```python
from build123d import *

# Parameters (mm, degrees)
F1_DEPTH = 20
F3_D     = 6
F4_SIZE  = 2
F5_R     = 2
F7_D     = 12
F7_DEPTH = 12
F7_TIP   = 3.6051637142
F9_D     = 12
F9_DEPTH = 12
F9_TIP   = 3.6051637142


# Not quite as in the source:
# - a feature names something its author has since deleted; it is built from what else it names


with BuildPart() as f1:
    # F0 (on Top) → F1 (new body)
    with BuildSketch(Plane.XY):
        with BuildLine():
            Line((0, 18), (0, 22.5))
            Line((0, 22.5), (0, 37.4649850279))
            Line((0, 37.4649850279), (-7, 37.4649850279))
            Line((-7, 37.4649850279), (-7, 24))
            ThreePointArc((-7, 24), (-25, 0), (-7, -24))
            Line((-7, -24), (-7, -37.4649850279))
            Line((-7, -37.4649850279), (0, -37.4649850279))
            Line((0, -37.4649850279), (0, -22.5))
            Line((0, -22.5), (0, -18))
            ThreePointArc((0, -18), (-18, 0), (0, 18))
        make_face()
    extrude(amount=F1_DEPTH)

    # F3 (through all)
    with Locations(Plane.YZ):
        with Locations((-30.75, 10), (30.75, 10)):
            Hole(F3_D / 2)

    # F4
    f4_edges = [f1.edges().sort_by_distance(p)[0] for p in [
        (-3.5, -37.464985, 20),
        (-3.5, -37.464985, 0),
        (-3.5, 37.464985, 20),
        (-3.5, 37.464985, 0),
    ]]
    chamfer(f4_edges, length=F4_SIZE)

    # F5
    f5_edges = [f1.edges().sort_by_distance(p)[0] for p in [
        (-7, -24, 10),
        (-7, 24, 10),
    ]]
    fillet(f5_edges, radius=F5_R)

    # F7 (one way)
    with BuildSketch(Plane(origin=(-7, 0, 0), x_dir=(0, -1, 0), z_dir=(1, 0, 0))):
        with Locations((30.75, -10)):
            Circle(F7_D / 2)
    extrude(amount=-F7_DEPTH, mode=Mode.SUBTRACT)
    with Locations(Plane(origin=(-7, 0, 0), x_dir=(0, -1, 0), z_dir=(1, 0, 0))):
        with Locations((30.75, -10)):
            with Locations((0, 0, -(F7_DEPTH + F7_TIP / 2))):  # 118° drill point
                Cone(0, F7_D / 2, F7_TIP, mode=Mode.SUBTRACT)

    # F9 (one way)
    with BuildSketch(Plane(origin=(-7, 0, 0), x_dir=(0, -1, 0), z_dir=(1, 0, 0))):
        with Locations((-30.75, -10)):
            Circle(F9_D / 2)
    extrude(amount=-F9_DEPTH, mode=Mode.SUBTRACT)
    with Locations(Plane(origin=(-7, 0, 0), x_dir=(0, -1, 0), z_dir=(1, 0, 0))):
        with Locations((-30.75, -10)):
            with Locations((0, 0, -(F9_DEPTH + F9_TIP / 2))):  # 118° drill point
                Cone(0, F9_D / 2, F9_TIP, mode=Mode.SUBTRACT)


solid = f1.part
```
Build history of the part. All positions in model axes, mm. Coordinates: 2 decimals unless noted, no trailing zeros. Order: outer loops, then holes, each group sorted by start corner. A loop starts at its lowest first (then second) coordinate and runs counter-clockwise, first axis right, second up. Notation, with made-up numbers: M -21.75,-24 L 28.25,-24 A10 cw 28.25,-6 Z; hole C -18,84.25 d11. An arc over 180 degrees is marked long. One line per question, with ' | ' between items. Start each with the question number.
1. Cut at A-A (z = 10). Write the cut outline in (x, y), plus the area to 3 significant figures.
2. Cut at C-C (y = 30.75). Write the cut outline in (x, z), plus the area to 3 significant figures.
3. Mould opens along Z. For faces 1 (the face through (-3.451, 36.479, 1.014)), 2 (the face through (-7.357, 24.315, 10.14)), 3 (the face through (-3.549, -36.479, 18.986)), 4 (the face through (-3.549, 33.747, 10.132)) say: +Z half, -Z half, draft (parallel to the pull), parting line (faces both ways), or undercut.
4. Cut at D-D (z = 13.75). Write the cut outline in (x, y), plus the area to 3 significant figures.
5. Wall check: line 1 along Z through (x, y) = (-2.25, -30.75); line 2 along Y through (x, z) = (-4.25, 10.75); line 3 along X through (y, z) = (31, 18.5). Give the ranges that are in metal, low to high. Write a range as [from, to].
6. Flat gauge pins, fed straight in: P1, Ø1, axis at y = 7.5, z = 7.5, coming from the +X side; P2, Ø9.5, axis at y = -30.75, z = 10, coming from the -X side; P3, Ø3, axis at x = -11.5, z = 6, coming from the -Y side; P4, Ø5, axis at y = 30.75, z = 10, coming from the -X side. Where does each tip first touch, or does it go through?
7. Cut at B-B (x = -1.25). Write the cut outline in (y, z).
The answers:
1) outline: M -8.33,-23.57 A2 cw -7.13,-24.75 L -7,-24.75 L -7,-27.75 L 0,-27.75 L 0,-18 A18 cw 0,18 L 0,27.75 L -7,27.75 L -7,24.75 L -7.13,24.75 A2 cw -8.33,23.57 A25 ccw Z; M -7,-37.46 L 0,-37.46 L 0,-33.75 L -7,-33.75 Z; M -7,33.75 L 0,33.75 L 0,37.46 L -7,37.46 Z | area: 569 mm2
2) outline: M -7,0 L 0,0 L 0,7 L -7,7 Z; M -7,13 L 0,13 L 0,20 L -7,20 Z | area: 98.0 mm2
3) face 1: -Z half | face 2: draft | face 3: +Z half | face 4: undercut
4) outline: M -8.33,-23.57 A2 cw -7,-25.46 L -7,-37.46 L 0,-37.46 L 0,-18 A18 cw 0,18 L 0,37.46 L -7,37.46 L -7,25.46 A2 cw -8.33,23.57 A25 ccw Z | area: 653 mm2
5) line 1: z = [0, 7], [13, 20] | line 2: y = [-37.46, -33.65], [-27.85, -17.49], [17.49, 27.85], [33.65, 37.46] | line 3: x = [-7, 0]
6) P1: stops at x = -16.12 | P2: stops at x = -7 | P3: stops at y = -22.91 | P4: passes through
7) outline: M -37.46,2 L -35.46,0 L -17.96,0 L -17.96,20 L -35.46,20 L -37.46,18 Z; M 17.96,0 L 35.46,0 L 37.46,2 L 37.46,18 L 35.46,20 L 17.96,20 Z; hole C -30.75,10 d6; hole C 30.75,10 d6
